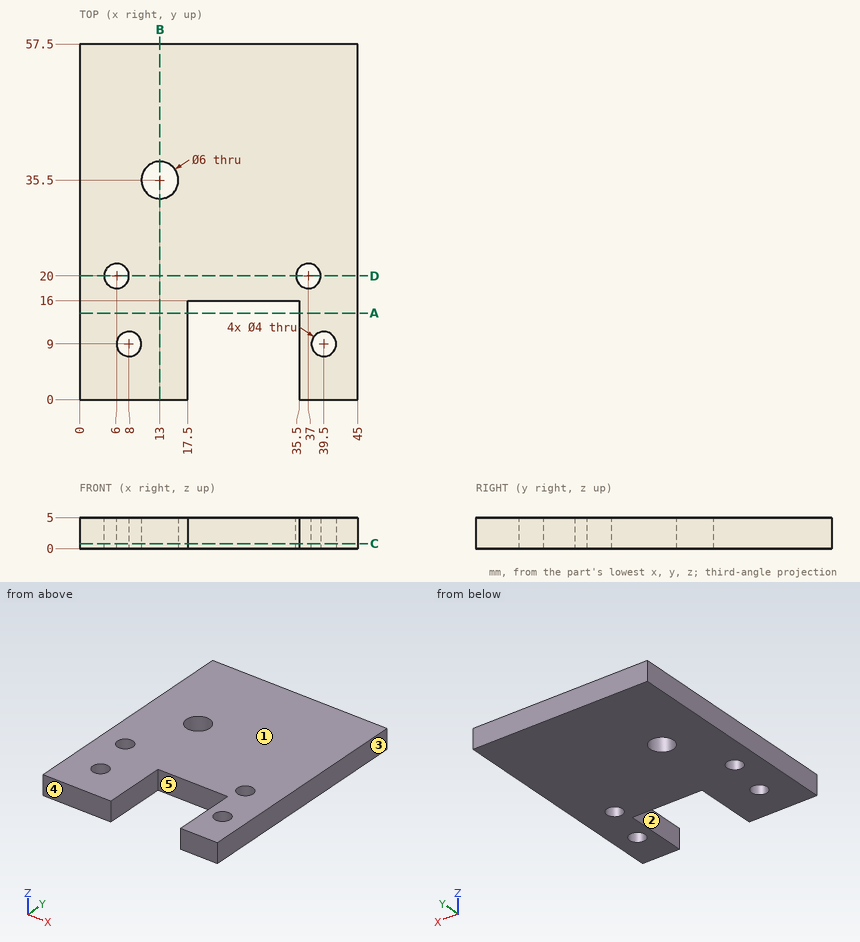
The drawing under review shows one solid part. Ordinate dimensions are in mm from its lowest x, y, z. A direction names the side the tool comes from. Give positions to 0.01 mm unless a question says otherwise; leave off trailing zeros. Order: outer loops, then holes, each group sorted by start corner. A loop starts at its lowest first (then second) coordinate and runs counter-clockwise, first axis right, second up. Notation, with made-up numbers: (3.25, -39.5) - (18.25, -39.5) arc R23 cw to (18.25, -24.5) - close; hole circle Ø3 at (79, 51). An arc over 180 degrees is marked (long way). Answer as a JSON object with one key per item and string values. Group by question number.
Item 1: Take a section at D-D on y = 20. Give the boundary of the cut face in (x, z), and give its area (3 significant figures).
Item 2: Wall thickness on line 1 along Y through (x, z) = (39.5, 0.45); line 2 along X through (y, z) = (3.5, 1.5); line 3 along Y through (x, z) = (18, 0.4): over which ranges is each line inside the solid? List them lowest first.
Item 3: Take a section at B-B on x = 13. Give the boundary of the cut face in (y, z), and give its area (4 significant figures).
Item 4: Take a section at C-C on z = 0.8. Give the boundary of the cut face in (x, y), and give its area (3 significant figures).
Item 5: Draft analysis for pull direction X (two halves, no side actions). For the marked faces 3, 4 and 5, state which applies: pulls with the +X half, pulls with the -X half, needs draft (parallel to the pull), parting line crosses it, or undercut.
Item 6: Machinability: for the marked faces 1 and 2, which of the approach directions +Z, -Z, +X, -X, +Y, -Y give a long, thin tool a straight path to every point of the face, cutting with its end or side? Answer none if there is none.
Item 7: Take a section at A-A on y = 14. Give the boundary of the cut face in (x, z).
Reported:
{
 "1": {"outline": "(0, 0) - (4, 0) - (4, 5) - (0, 5) - close; (8, 0) - (35, 0) - (35, 5) - (8, 5) - close; (39, 0) - (45, 0) - (45, 5) - (39, 5) - close", "area": "185 mm^2"},
 "2": {"line 1": "0 to 7, 11 to 57.5", "line 2": "0 to 17.5, 35.5 to 45", "line 3": "16 to 57.5"},
 "3": {"outline": "(0, 0) - (32.5, 0) - (32.5, 5) - (0, 5) - close; (38.5, 0) - (57.5, 0) - (57.5, 5) - (38.5, 5) - close", "area": "257.5 mm^2"},
 "4": {"outline": "(0, 0) - (17.5, 0) - (17.5, 16) - (35.5, 16) - (35.5, 0) - (45, 0) - (45, 57.5) - (0, 57.5) - close; hole circle Ø4 at (6, 20); hole circle Ø4 at (8, 9); hole circle Ø6 at (13, 35.5); hole circle Ø4 at (37, 20); hole circle Ø4 at (39.5, 9)", "area": "2,220 mm^2"},
 "5": {"face 3": "pulls with the +X half", "face 4": "needs draft", "face 5": "undercut"},
 "6": {"face 1": "+Z, +X, -X, +Y, -Y", "face 2": "+Z, -Z, -Y"},
 "7": {"outline": "(0, 0) - (17.5, 0) - (17.5, 5) - (0, 5) - close; (35.5, 0) - (45, 0) - (45, 5) - (35.5, 5) - close"}
}
